The model under review builds one solid part; all positions refer to its coordinate system, in mm. A direction names the side the tool comes from. Round coordinates to 2 decimals unless told otherwise and drop trailing zeros. Order: outer loops, then holes, each group sorted by start corner. A loop starts at its lowest first (then second) coordinate and runs counter-clockwise, first axis right, second up. Notation, with made-up numbers: (84.5, 84) -> (120.5, 84) arc R23 cw to (120.5, 119) -> close; hole circle Ø1 at (11.5, 82.25). An arc over 180 degrees is marked (long way). Use a Markdown table: item, result. Add a question column.
```python
from build123d import *

# Parameters (mm, degrees)
SKETCH1_W               = 95
SKETCH1_H               = 32
BASE_FLANGE1_DEPTH      = 3.5
EDGE_FLANGE1_DEPTH      = 32
EDGE_FLANGE1_BEND_DEPTH = 32
EDGE_FLANGE2_DEPTH      = 32
EDGE_FLANGE2_BEND_DEPTH = 32
EDGE_FLANGE3_DEPTH      = 8
EDGE_FLANGE4_DEPTH      = 32
SKETCH30_R              = 6.5
SKETCH30_R_2            = 4
SKETCH30_W              = 20.215069336
SKETCH30_H              = 12
CUT_EXTRUDE1_DEPTH      = 10
CUT_EXTRUDE2_OUTLINE_W  = 31.867862703
CUT_EXTRUDE2_OUTLINE_H  = 3.5
CUT_EXTRUDE2_DEPTH      = 14
CUT_EXTRUDE2_2_DEPTH    = 10


# Read off the part's stored shape, not the designer's step: Cut-Extrude2
# Sheet-metal steps are written as plain solids
with BuildPart() as part:
    # Sketch1 → Base-Flange1 (new body)
    with BuildSketch(Plane(origin=(0, 0, 0), x_dir=(1, 0, 0), z_dir=(0, 1, 0))):
        Rectangle(SKETCH1_W, SKETCH1_H)
    extrude(amount=-BASE_FLANGE1_DEPTH)

    # Edge-Flange1 section (across the edge) → Edge-Flange1 (add)
    with BuildSketch(Plane(origin=(48.5, -3.5, -16), x_dir=(-1, 0, 0), z_dir=(0, 0, 1))):
        with BuildLine():
            Line((-3.5, 1), (-3.5, 41))
            Line((-3.5, 41), (0, 41))
            Line((0, 41), (0, 1))
            ThreePointArc((0, 1), (0.292893219, 0.292893219), (1, 0))
            Line((1, 0), (1, -3.5))
            ThreePointArc((1, -3.5), (-2.181980515, -2.181980515), (-3.5, 1))
        make_face()
    extrude(amount=EDGE_FLANGE1_DEPTH)

    # Edge-Flange1 section 2 (across the edge) → Edge-Flange1 bend (add)
    with BuildSketch(Plane(origin=(-48.5, -3.5, 16), x_dir=(1, 0, 0), z_dir=(0, 0, -1))):
        with BuildLine():
            Line((-3.5, 1), (-3.5, 41))
            Line((-3.5, 41), (0, 41))
            Line((0, 41), (0, 1))
            ThreePointArc((0, 1), (0.292893219, 0.292893219), (1, 0))
            Line((1, 0), (1, -3.5))
            ThreePointArc((1, -3.5), (-2.181980515, -2.181980515), (-3.5, 1))
        make_face()
    extrude(amount=EDGE_FLANGE1_BEND_DEPTH)

    # Edge-Flange2 section (across the edge) → Edge-Flange2 (add)
    with BuildSketch(Plane(origin=(52, -45.5, 16), x_dir=(0, 1, 0), z_dir=(0, 0, -1))):
        with BuildLine():
            Line((-3.5, 1), (-3.5, 22))
            Line((-3.5, 22), (0, 22))
            Line((0, 22), (0, 1))
            ThreePointArc((0, 1), (0.292893219, 0.292893219), (1, 0))
            Line((1, 0), (1, -3.5))
            ThreePointArc((1, -3.5), (-2.181980515, -2.181980515), (-3.5, 1))
        make_face()
    extrude(amount=EDGE_FLANGE2_DEPTH)

    # Edge-Flange2 section 2 (across the edge) → Edge-Flange2 bend (add)
    with BuildSketch(Plane(origin=(-52, -45.5, -16), x_dir=(0, 1, 0), z_dir=(0, 0, 1))):
        with BuildLine():
            Line((-3.5, 1), (-3.5, 22))
            Line((-3.5, 22), (0, 22))
            Line((0, 22), (0, 1))
            ThreePointArc((0, 1), (0.292893219, 0.292893219), (1, 0))
            Line((1, 0), (1, -3.5))
            ThreePointArc((1, -3.5), (-2.181980515, -2.181980515), (-3.5, 1))
        make_face()
    extrude(amount=EDGE_FLANGE2_BEND_DEPTH)

    # Edge-Flange3 section (across the edge) → Edge-Flange3 (add)
    with BuildSketch(Plane(origin=(-2, -3.5, 17), x_dir=(0, 0, -1), z_dir=(-1, 0, 0))):
        with BuildLine():
            Line((-3.5, 1), (-3.5, 19))
            Line((-3.5, 19), (0, 19))
            Line((0, 19), (0, 1))
            ThreePointArc((0, 1), (0.292893219, 0.292893219), (1, 0))
            Line((1, 0), (1, -3.5))
            ThreePointArc((1, -3.5), (-2.181980515, -2.181980515), (-3.5, 1))
        make_face()
    extrude(amount=EDGE_FLANGE3_DEPTH)

    # Edge-Flange4 section (across the edge) → Edge-Flange4 (add)
    with BuildSketch(Plane(origin=(32, -3.5, 17), x_dir=(0, 0, -1), z_dir=(-1, 0, 0))):
        with BuildLine():
            Line((-3.5, 1), (-3.5, 44))
            Line((-3.5, 44), (0, 44))
            Line((0, 44), (0, 1))
            ThreePointArc((0, 1), (0.292893219, 0.292893219), (1, 0))
            Line((1, 0), (1, -3.5))
            ThreePointArc((1, -3.5), (-2.181980515, -2.181980515), (-3.5, 1))
        make_face()
    extrude(amount=EDGE_FLANGE4_DEPTH)

    # Sketch30 → Cut-Extrude1 (cut)
    # profile 1 of 2: a face of its own
    with BuildSketch(Plane(origin=(0, 0, 0), x_dir=(1, 0, 0), z_dir=(0, 1, 0))):
        with Locations(Location((36.215069336, -6, 0), (0, 0, 270))):
            Circle(SKETCH30_R)
        with Locations((36.215069336, -6)):
            Circle(SKETCH30_R_2, mode=Mode.SUBTRACT)
    # profile 2 of 2: a face of its own
    with BuildSketch(Plane(origin=(0, 0, 0), x_dir=(1, 0, 0), z_dir=(0, 1, 0))):
        with Locations((8.107534668, -10)):
            Rectangle(SKETCH30_W, SKETCH30_H)
    extrude(amount=-CUT_EXTRUDE1_DEPTH, mode=Mode.SUBTRACT)


with BuildPart() as cut_extrude1_kept_piece:
    # of the separate pieces the step leaves, the one the design keeps (cut_extrude1_pieces_kept)
    add(part.part.solids().sort_by_distance((-47.5, -3.5, -16))[0])

    # Cut-Extrude2 outline → Cut-Extrude2 (cut)
    with BuildSketch(Plane.YZ):
        with Locations((-31.566068648, 18.75)):
            Rectangle(CUT_EXTRUDE2_OUTLINE_W, CUT_EXTRUDE2_OUTLINE_H)
    extrude(amount=CUT_EXTRUDE2_DEPTH, mode=Mode.SUBTRACT)

    # Cut-Extrude2 2 outline → Cut-Extrude2 2 (cut)
    with BuildSketch(Plane.YZ):
        with BuildLine():
            Line((-9, 20.5), (-9, 17))
            Line((-9, 17), (-4.5, 17))
            ThreePointArc((-4.5, 17), (-3.841719411, 16.752772652), (-3.50892875, 16.133333333))
            Line((-3.50892875, 16.133333333), (-0.040179376, 16.6))
            ThreePointArc((-0.040179376, 16.6), (-1.537737352, 19.387476937), (-4.5, 20.5))
            Line((-4.5, 20.5), (-9, 20.5))
        make_face()
    extrude(amount=CUT_EXTRUDE2_2_DEPTH, mode=Mode.SUBTRACT)


solid = cut_extrude1_kept_piece.part
```
Q1. Machinability: for faces 4 (the flat face through (-1, -3.5, 0)), 5 (the flat face through (18.215, -2, 10)), 6 (the flat face through (-48.5, -25, 0)), 7 (the flat face through (-2, -7.9, 17.2)), which of the approach directions +Z, -Z, +X, -X, +Y, -Y give a long, thin tool a straight path to every point of the face, cutting with its end or side? Answer none if there is none.
Q2. Add section B-B (y = -7). Write out the cut boundary in (x, z).
Q3. Add section A-A (z = 6). Write out the cut boundary in (x, y).
Q4. Insertion check: pin 1 (4 mm diameter, centred on y = -37, z = 5.5, fed in from +X); pin 2 (4 mm diameter, centred on x = -3.5, y = -8.5, fed in from -Z); pin 3 (5 mm diameter, centred on y = -12.5, z = 19, fed in from -X); pin 4 (11.5 mm diameter, centred on x = 36.22, z = 6, fed in from -Y). Each pin has a flat end and moves straight along its axis. Give the tip position at first contact, or say it passes through.
Q5. Mouldability with a two-part tool opening along X and no side actions: class faces 1 (the cylindrical face through (49.783, -47.647, 0.224)), 2 (the flat face through (74, -47, 0)), 3 (the flat face through (23, -26, 17)) as pulls with the +X half, pulls with the -X half, needs draft (parallel to the pull), parting line crosses it, or undercut.
Q6. Wall thickness on line 1 (X direction, y = -6, z = 3.5); line 2 (X direction, y = -2, z = 6); line 3 (Z direction, x = 51, y = -14): over which ranges is each line inside the solid? List them lowest first. Write a range as [from, to].
Q7. Add section C-C (y = -40.5). Write out the cut boundary in (x, z), then the cut area to 3 significant figures.
Q8. Add section D-D (x = -58). Write out the cut boundary in (y, z).
Report:
| question | item | result |
|---|---|---|
| 1 | face 4 | -Z, -Y |
| 1 | face 5 | +Y, -Y |
| 1 | face 6 | +Z, -Z, -Y |
| 1 | face 7 | +Z, +Y, -Y |
| 2 | outline | (-52, -16) -> (-48.5, -16) -> (-48.5, 16) -> (-52, 16) -> close; (-10, 17) -> (-2, 17) -> (-2, 20.5) -> (-10, 20.5) -> close; (10, 17) -> (32, 17) -> (32, 20.5) -> (10, 20.5) -> close; (48.5, -16) -> (52, -16) -> (52, 16) -> (48.5, 16) -> close |
| 3 | outline | (-74, -49) -> (-53, -49) arc R4.5 ccw to (-48.5, -44.5) -> (-48.5, -4.5) arc R1 cw to (-47.5, -3.5) -> (-2, -3.5) -> (-2, 0) -> (-47.5, 0) arc R4.5 ccw to (-52, -4.5) -> (-52, -44.5) arc R1 cw to (-53, -45.5) -> (-74, -45.5) -> close; (18.22, -3.5) -> (29.72, -3.5) -> (29.72, 0) -> (18.22, 0) -> close; (42.72, -3.5) -> (47.5, -3.5) arc R1 cw to (48.5, -4.5) -> (48.5, -44.5) arc R4.5 ccw to (53, -49) -> (74, -49) -> (74, -45.5) -> (53, -45.5) arc R1 cw to (52, -44.5) -> (52, -4.5) arc R4.5 ccw to (47.5, 0) -> (42.72, 0) -> close |
| 4 | pin 1 | stops at x = 52 |
| 4 | pin 2 | stops at z = 17 |
| 4 | pin 3 | stops at x = -10 |
| 4 | pin 4 | passes through |
| 5 | face 1 | undercut |
| 5 | face 2 | pulls with the +X half |
| 5 | face 3 | needs draft |
| 6 | line 1 | x = [-52, -48.5], [48.5, 52] |
| 6 | line 2 | x = [-51.24, -2], [18.22, 29.72], [42.72, 51.24] |
| 6 | line 3 | z = [-16, 16] |
| 7 | outline | (-52, -16) -> (-48.5, -16) -> (-48.5, 16) -> (-52, 16) -> close; (14, 17) -> (32, 17) -> (32, 20.5) -> (14, 20.5) -> close; (48.5, -16) -> (52, -16) -> (52, 16) -> (48.5, 16) -> close |
| 7 | area | 287 mm² |
| 8 | outline | (-49, -16) -> (-45.5, -16) -> (-45.5, 16) -> (-49, 16) -> close |
